from build123d import *

# Parameters (mm, degrees)
F1_DEPTH = 6


with BuildPart() as f1:
    # F0 (on Top) → F1 (new body)
    with BuildSketch(Plane.XY):
        with BuildLine():
            Line((-4.3394552469, -10.0690543538), (-4.3394552469, -2.0690543538))
            Line((-4.3394552469, -2.0690543538), (-16.3394552469, -2.0690543538))
            ThreePointArc((-16.3394552469, -2.0690543538), (-16.9252416846, -3.4832679161), (-18.3394552469, -4.0690543538))
            ThreePointArc((-18.3394552469, -4.0690543538), (-19.7536688093, -3.4832679161), (-20.3394552469, -2.0690543538))
            Line((-20.3394552469, -2.0690543538), (-29.3394552469, -2.0690543538))
            ThreePointArc((-29.3394552469, -2.0690543538), (-32.3394552469, -5.0690543538), (-35.3394552469, -2.0690543538))
            Line((-35.3394552469, -2.0690543538), (-41.3394552469, -2.0690543538))
            Line((-41.3394552469, -2.0690543538), (-41.3394552469, -5.0690543538))
            Line((-41.3394552469, -5.0690543538), (-41.3394552469, -10.0690543538))
            Line((-41.3394552469, -10.0690543538), (-36.3394552469, -10.0690543538))
            Line((-36.3394552469, -10.0690543538), (-13.5731431865, -10.0690543538))
            Line((-13.5731431865, -10.0690543538), (-13.1868220354, -10.0690543538))
            Line((-13.1868220354, -10.0690543538), (-4.3394552469, -10.0690543538))
        make_face()
        with BuildLine():
            Line((-4.3394552469, 5.9309456462), (-4.3394552469, -2.0690543538))
            ThreePointArc((-4.3394552469, -2.0690543538), (-1.9963094964, 3.5877998957), (3.6605447531, 5.9309456462))
            Line((3.6605447531, 5.9309456462), (-4.3394552469, 5.9309456462))
        make_face()
        with BuildLine():
            ThreePointArc((3.6605447531, -10.0690543538), (-1.9963094964, -7.7259086033), (-4.3394552469, -2.0690543538))
            Line((-4.3394552469, -2.0690543538), (-4.3394552469, -10.0690543538))
            Line((-4.3394552469, -10.0690543538), (3.6605447531, -10.0690543538))
        make_face()
        with BuildLine():
            Line((-16.3394552469, -2.0690543538), (-4.3394552469, -2.0690543538))
            Line((-4.3394552469, -2.0690543538), (-4.3394552469, 5.9309456462))
            Line((-4.3394552469, 5.9309456462), (-11.6972615942, 5.9309456462))
            Line((-11.6972615942, 5.9309456462), (-13.5731431865, 5.9309456462))
            Line((-13.5731431865, 5.9309456462), (-36.3394552469, 5.9309456462))
            Line((-36.3394552469, 5.9309456462), (-41.3394552469, 5.9309456462))
            Line((-41.3394552469, 5.9309456462), (-41.3394552469, 0.9309456462))
            Line((-41.3394552469, 0.9309456462), (-41.3394552469, -2.0690543538))
            Line((-41.3394552469, -2.0690543538), (-35.3394552469, -2.0690543538))
            ThreePointArc((-35.3394552469, -2.0690543538), (-34.4607755905, 0.0522659898), (-32.3394552469, 0.9309456462))
            ThreePointArc((-32.3394552469, 0.9309456462), (-30.2181349034, 0.0522659898), (-29.3394552469, -2.0690543538))
            Line((-29.3394552469, -2.0690543538), (-20.3394552469, -2.0690543538))
            ThreePointArc((-20.3394552469, -2.0690543538), (-18.3394552469, -0.0690543538), (-16.3394552469, -2.0690543538))
        make_face()
        with BuildLine():
            Line((11.6605447531, 5.9309456462), (3.6605447531, 5.9309456462))
            ThreePointArc((3.6605447531, 5.9309456462), (9.3173990026, 3.5877998957), (11.6605447531, -2.0690543538))
            Line((11.6605447531, -2.0690543538), (11.6605447531, 5.9309456462))
        make_face()
        with BuildLine():
            Line((-4.3394552469, 5.9309456462), (3.6605447531, 5.9309456462))
            Line((3.6605447531, 5.9309456462), (3.6605447531, 17.9309456462))
            ThreePointArc((3.6605447531, 17.9309456462), (1.6605447531, 19.9309456462), (3.6605447531, 21.9309456462))
            Line((3.6605447531, 21.9309456462), (3.6605447531, 31.9309456462))
            ThreePointArc((3.6605447531, 31.9309456462), (0.6605447531, 34.9309456462), (3.6605447531, 37.9309456462))
            Line((3.6605447531, 37.9309456462), (3.6605447531, 42.9309456462))
            Line((3.6605447531, 42.9309456462), (0.6605447531, 42.9309456462))
            Line((0.6605447531, 42.9309456462), (-4.3394552469, 42.9309456462))
            Line((-4.3394552469, 42.9309456462), (-4.3394552469, 37.9309456462))
            Line((-4.3394552469, 37.9309456462), (-4.3394552469, 15.1646335859))
            Line((-4.3394552469, 15.1646335859), (-4.3394552469, 14.7783124347))
            Line((-4.3394552469, 14.7783124347), (-4.3394552469, 5.9309456462))
        make_face()
        with BuildLine():
            Line((3.6605447531, 17.9309456462), (3.6605447531, 5.9309456462))
            Line((3.6605447531, 5.9309456462), (11.6605447531, 5.9309456462))
            Line((11.6605447531, 5.9309456462), (11.6605447531, 13.2887519935))
            Line((11.6605447531, 13.2887519935), (11.6605447531, 15.1646335859))
            Line((11.6605447531, 15.1646335859), (11.6605447531, 37.9309456462))
            Line((11.6605447531, 37.9309456462), (11.6605447531, 42.9309456462))
            Line((11.6605447531, 42.9309456462), (6.6605447531, 42.9309456462))
            Line((6.6605447531, 42.9309456462), (3.6605447531, 42.9309456462))
            Line((3.6605447531, 42.9309456462), (3.6605447531, 37.9309456462))
            ThreePointArc((3.6605447531, 37.9309456462), (5.7818650966, 37.0522659898), (6.6605447531, 34.9309456462))
            ThreePointArc((6.6605447531, 34.9309456462), (5.7818650966, 32.8096253027), (3.6605447531, 31.9309456462))
            Line((3.6605447531, 31.9309456462), (3.6605447531, 21.9309456462))
            ThreePointArc((3.6605447531, 21.9309456462), (5.0747583154, 21.3451592086), (5.6605447531, 19.9309456462))
            ThreePointArc((5.6605447531, 19.9309456462), (5.0747583154, 18.5167320839), (3.6605447531, 17.9309456462))
        make_face()
        with BuildLine():
            Line((11.6605447531, -10.0690543538), (3.6605447531, -10.0690543538))
            Line((3.6605447531, -10.0690543538), (3.6605447531, -22.0690543538))
            ThreePointArc((3.6605447531, -22.0690543538), (5.0747583154, -22.6548407914), (5.6605447531, -24.0690543538))
            ThreePointArc((5.6605447531, -24.0690543538), (5.0747583154, -25.4832679161), (3.6605447531, -26.0690543538))
            Line((3.6605447531, -26.0690543538), (3.6605447531, -36.0690543538))
            ThreePointArc((3.6605447531, -36.0690543538), (5.7818650966, -36.9477340102), (6.6605447531, -39.0690543538))
            ThreePointArc((6.6605447531, -39.0690543538), (5.7818650966, -41.1903746973), (3.6605447531, -42.0690543538))
            Line((3.6605447531, -42.0690543538), (3.6605447531, -47.0690543538))
            Line((3.6605447531, -47.0690543538), (6.6605447531, -47.0690543538))
            Line((6.6605447531, -47.0690543538), (11.6605447531, -47.0690543538))
            Line((11.6605447531, -47.0690543538), (11.6605447531, -42.0690543538))
            Line((11.6605447531, -42.0690543538), (11.6605447531, -19.3027422934))
            Line((11.6605447531, -19.3027422934), (11.6605447531, -18.9164211423))
            Line((11.6605447531, -18.9164211423), (11.6605447531, -10.0690543538))
        make_face()
        with BuildLine():
            Line((3.6605447531, -22.0690543538), (3.6605447531, -10.0690543538))
            Line((3.6605447531, -10.0690543538), (-4.3394552469, -10.0690543538))
            Line((-4.3394552469, -10.0690543538), (-4.3394552469, -17.4268607011))
            Line((-4.3394552469, -17.4268607011), (-4.3394552469, -19.3027422934))
            Line((-4.3394552469, -19.3027422934), (-4.3394552469, -42.0690543538))
            Line((-4.3394552469, -42.0690543538), (-4.3394552469, -45.6229187548))
            Line((-4.3394552469, -45.6229187548), (-4.3394552469, -47.0690543538))
            Line((-4.3394552469, -47.0690543538), (0.6605447531, -47.0690543538))
            Line((0.6605447531, -47.0690543538), (3.6605447531, -47.0690543538))
            Line((3.6605447531, -47.0690543538), (3.6605447531, -42.0690543538))
            ThreePointArc((3.6605447531, -42.0690543538), (0.6605447531, -39.0690543538), (3.6605447531, -36.0690543538))
            Line((3.6605447531, -36.0690543538), (3.6605447531, -26.0690543538))
            ThreePointArc((3.6605447531, -26.0690543538), (1.6605447531, -24.0690543538), (3.6605447531, -22.0690543538))
        make_face()
        with BuildLine():
            ThreePointArc((11.6605447531, -2.0690543538), (9.3173990026, -7.7259086033), (3.6605447531, -10.0690543538))
            Line((3.6605447531, -10.0690543538), (11.6605447531, -10.0690543538))
            Line((11.6605447531, -10.0690543538), (11.6605447531, -2.0690543538))
        make_face()
        with BuildLine():
            Line((11.6605447531, 5.9309456462), (11.6605447531, -2.0690543538))
            Line((11.6605447531, -2.0690543538), (23.6605447531, -2.0690543538))
            ThreePointArc((23.6605447531, -2.0690543538), (24.2463311907, -0.6548407914), (25.6605447531, -0.0690543538))
            ThreePointArc((25.6605447531, -0.0690543538), (27.0747583154, -0.6548407914), (27.6605447531, -2.0690543538))
            Line((27.6605447531, -2.0690543538), (37.6605447531, -2.0690543538))
            ThreePointArc((37.6605447531, -2.0690543538), (38.5392244095, 0.0522659898), (40.6605447531, 0.9309456462))
            ThreePointArc((40.6605447531, 0.9309456462), (42.7818650966, 0.0522659898), (43.6605447531, -2.0690543538))
            Line((43.6605447531, -2.0690543538), (48.6605447531, -2.0690543538))
            Line((48.6605447531, -2.0690543538), (48.6605447531, 0.9309456462))
            Line((48.6605447531, 0.9309456462), (48.6605447531, 5.9309456462))
            Line((48.6605447531, 5.9309456462), (43.6605447531, 5.9309456462))
            Line((43.6605447531, 5.9309456462), (20.8942326927, 5.9309456462))
            Line((20.8942326927, 5.9309456462), (20.5079115416, 5.9309456462))
            Line((20.5079115416, 5.9309456462), (11.6605447531, 5.9309456462))
        make_face()
        with BuildLine():
            Line((23.6605447531, -2.0690543538), (11.6605447531, -2.0690543538))
            Line((11.6605447531, -2.0690543538), (11.6605447531, -10.0690543538))
            Line((11.6605447531, -10.0690543538), (19.0183511004, -10.0690543538))
            Line((19.0183511004, -10.0690543538), (20.8942326927, -10.0690543538))
            Line((20.8942326927, -10.0690543538), (43.6605447531, -10.0690543538))
            Line((43.6605447531, -10.0690543538), (48.6605447531, -10.0690543538))
            Line((48.6605447531, -10.0690543538), (48.6605447531, -5.0690543538))
            Line((48.6605447531, -5.0690543538), (48.6605447531, -2.0690543538))
            Line((48.6605447531, -2.0690543538), (43.6605447531, -2.0690543538))
            ThreePointArc((43.6605447531, -2.0690543538), (40.6605447531, -5.0690543538), (37.6605447531, -2.0690543538))
            Line((37.6605447531, -2.0690543538), (27.6605447531, -2.0690543538))
            ThreePointArc((27.6605447531, -2.0690543538), (25.6605447531, -4.0690543538), (23.6605447531, -2.0690543538))
        make_face()
        Polygon((-4.3394552469, -17.4268607011), (-4.3394552469, -10.0690543538), (-13.1868220354, -10.0690543538), (-13.5731431865, -10.0690543538), (-8.9562992167, -14.6858983236), (-4.3394552469, -19.3027422934), align=None)
        Polygon((-11.6972615942, 5.9309456462), (-4.3394552469, 5.9309456462), (-4.3394552469, 14.7783124347), (-4.3394552469, 15.1646335859), (-8.9562992167, 10.547789616), (-13.5731431865, 5.9309456462), align=None)
        Polygon((11.6605447531, 13.2887519935), (11.6605447531, 5.9309456462), (20.5079115416, 5.9309456462), (20.8942326927, 5.9309456462), (16.2773887229, 10.547789616), (11.6605447531, 15.1646335859), align=None)
        Polygon((19.0183511004, -10.0690543538), (11.6605447531, -10.0690543538), (11.6605447531, -18.9164211423), (11.6605447531, -19.3027422934), (16.2773887229, -14.6858983236), (20.8942326927, -10.0690543538), align=None)
        Polygon((-4.3394552469, -42.0690543538), (-4.3394552469, -19.3027422934), (-8.9562992167, -14.6858983236), (-4.3394552469, -45.6229187548), align=None)
        Polygon((-8.9562992167, -14.6858983236), (-13.5731431865, -10.0690543538), (-36.3394552469, -10.0690543538), (-41.3394552469, -10.0690543538), align=None)
        Polygon((-8.9562992167, 10.547789616), (-4.3394552469, 15.1646335859), (-4.3394552469, 37.9309456462), (-4.3394552469, 42.9309456462), align=None)
        Polygon((-36.3394552469, 5.9309456462), (-13.5731431865, 5.9309456462), (-8.9562992167, 10.547789616), (-41.3394552469, 5.9309456462), align=None)
        Polygon((11.6605447531, 37.9309456462), (11.6605447531, 15.1646335859), (16.2773887229, 10.547789616), (11.6605447531, 42.9309456462), align=None)
        Polygon((16.2773887229, 10.547789616), (20.8942326927, 5.9309456462), (43.6605447531, 5.9309456462), (48.6605447531, 5.9309456462), align=None)
        Polygon((16.2773887229, -14.6858983236), (11.6605447531, -19.3027422934), (11.6605447531, -42.0690543538), (11.6605447531, -47.0690543538), align=None)
        Polygon((43.6605447531, -10.0690543538), (20.8942326927, -10.0690543538), (16.2773887229, -14.6858983236), (48.6605447531, -10.0690543538), align=None)
    extrude(amount=-F1_DEPTH)


solid = f1.part
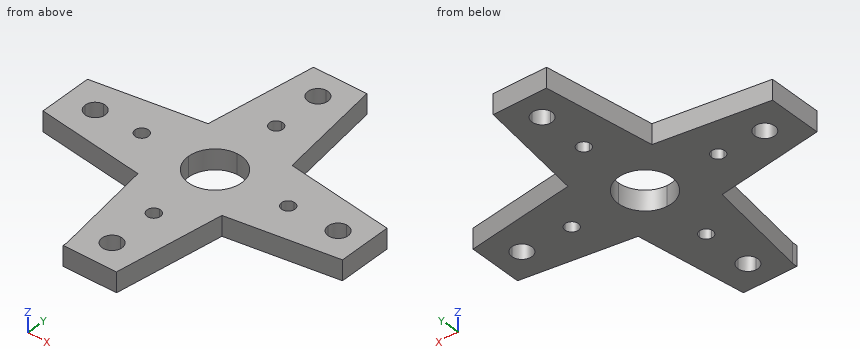
For this review, take the finished solid that the model builds, in its own axes (mm). Round coordinates to 2 decimals unless told otherwise and drop trailing zeros. Order: outer loops, then holes, each group sorted by start corner. A loop starts at its lowest first (then second) coordinate and runs counter-clockwise, first axis right, second up. Notation, with made-up numbers: M 11,60.5 L 23,60.5 A10 ccw 23,66.5 Z; hole C 35,15.25 d5. An arc over 180 degrees is marked long. Use a Markdown table: item, result. Add a question column.
Item 1: Add section D-D, the plane y = 12. Give the boundary of the cut face in (x, z), then the cut area to 3 significant figures.
Item 2: Add section C-C, the plane z = -4. State how many separate pieces and enclosed holes the cut face has, then the cut area to 3 significant figures.
Item 3: Add section A-A, the plane y = 3. Give the boundary of the cut face in (x, z), then the cut area to 3 significant figures.
Item 4: Insertion check: pin 1 (3 mm diameter, centred on x = -31, z = -2.5, fed in from +Y); pin 2 (0.7 mm diameter, centred on y = -46.5, z = -1.5, fed in from -X); pin 3 (1 mm diameter, centred on x = -17.5, z = -4, fed in from +Y). Each pin has a flat end and moves straight along its axis. Give the tip position at first contact, or say it passes through.
Item 5: To check wall thickness, follow line 1 along X through (y, z) = (0, -0.2); line 2 along Y through (x, z) = (9, -5.05); line 3 along X through (y, z) = (2, -4.55). State the ranges of each line that lie inside material, in increasing order.
Item 6: Add section B-B, the plane x = -2.5. Give the boundary of the cut face in (y, z), then the cut area to 3 significant figures.
Geometry results:
| question | item | result |
|---|---|---|
| 1 | outline | M -8.75,-6 L 16.07,-6 L 16.07,0 L -8.75,0 Z |
| 1 | area | 149 mm² |
| 2 | separate pieces | 1 |
| 2 | enclosed holes | 9 |
| 2 | area | 2,940 mm² |
| 3 | outline | M -41.34,-6 L -2.53,-6 L -2.53,0 L -41.34,0 Z; M 9.85,-6 L 48.66,-6 L 48.66,0 L 9.85,0 Z |
| 3 | area | 466 mm² |
| 4 | pin 1 | stops at y = 7.62 |
| 4 | pin 2 | stops at x = -4.34 |
| 4 | pin 3 | stops at y = 9.4 |
| 5 | line 1 | x = -41.34 to -34.51, -30.17 to -4.07, 11.39 to 38.49, 42.83 to 48.66 |
| 5 | line 2 | y = -47.07 to -8.03, 3.89 to 42.93 |
| 5 | line 3 | x = -41.34 to -3.23, 10.55 to 48.66 |
| 6 | outline | M -47.07,-6 L -7.17,-6 L -7.17,0 L -47.07,0 Z; M 3.03,-6 L 42.93,-6 L 42.93,0 L 3.03,0 Z |
| 6 | area | 479 mm² |
